Input: part model. Units: mm. Frame: model coordinates. A direction names the side the tool comes from. Coordinates: 2 decimals unless noted, no trailing zeros. Write each loop counter-clockwise with the first axis right and the second up, starting at its lowest first coordinate (ties: lowest second). Pieces come first, ordered by that corner, then holes.
from build123d import *

# Parameters (mm, degrees)
BOSS_EXTRUDE1_DEPTH     = 30
SKETCH2_W               = 30
SKETCH2_H               = 30
CUT_EXTRUDE1_DEPTH      = 30
CHAMFER1_SIZE           = 3
FILLET1_R               = 3
FILLET2_R               = 3
CUT_EXTRUDE2_DEPTH      = 30
CUT_EXTRUDE2_DEPTH_BACK = 30
SKETCH3_R               = 1.75
CUT_EXTRUDE3_DEPTH      = 50
CUT_EXTRUDE3_DEPTH_BACK = 30
SKETCH4_R               = 3
CUT_EXTRUDE4_DEPTH      = 88.933914818
CUT_EXTRUDE4_DEPTH_BACK = 88.933914818
SKETCH5_R               = 1.75


with BuildPart() as part:
    # Sketch1 → Boss-Extrude1 (new body)
    with BuildSketch(Plane(origin=(0, 0, 0), x_dir=(1, 0, 0), z_dir=(0, 1, 0))):
        Polygon((-65, 21.062445841), (-65, -21.062445841), (-21.005807434, -21.062445841), (-21.005807434, -30), (-15, -30), (-15, -21.062445841), (-36.062445841, 0), (-15, 21.062445841), (-15, 30), (-22, 30), (-22, 21.062445841), align=None)
    extrude(amount=BOSS_EXTRUDE1_DEPTH)

    # Sketch2 → Cut-Extrude1 (cut)
    with BuildSketch(Plane(origin=(0, 30, 0), x_dir=(1, 0, 0), z_dir=(0, 1, 0))):
        with Locations((-56.062445841, 0)):
            Rectangle(SKETCH2_W, SKETCH2_H)
    extrude(amount=-CUT_EXTRUDE1_DEPTH, mode=Mode.SUBTRACT)

    # Chamfer1
    chamfer1_edges = [part.edges().sort_by_distance(p)[0] for p in [
        (-21.005807434, 15, 21.062445841),
        (-22, 15, -21.062445841),
    ]]
    chamfer(chamfer1_edges, length=CHAMFER1_SIZE)

    # Fillet1
    fillet1_edges = [part.edges().sort_by_distance(p)[0] for p in [
        (-36.062445841, 15, 0),
        (-15, 15, 21.062445841),
        (-15, 15, -21.062445841),
        (-41.062445841, 15, 15),
        (-41.062445841, 15, -15),
    ]]
    fillet(fillet1_edges, radius=FILLET1_R)

    # Fillet2
    fillet2_edges = [part.edges().sort_by_distance(p)[0] for p in [
        (-15, 15, 30),
        (-21.005807434, 15, 30),
        (-65, 15, 21.062445841),
        (-65, 15, -21.062445841),
        (-22, 15, -30),
        (-15, 15, -30),
        (-65, 15, 15),
        (-65, 15, -15),
    ]]
    fillet(fillet2_edges, radius=FILLET2_R)

    # Sketch3 → Cut-Extrude2 (cut, two sides: drawn at the far end of the back side and taken through both)
    with BuildSketch(Plane.ZY.offset(22).offset(-CUT_EXTRUDE2_DEPTH_BACK)):
        with Locations(Location((-25, 15, 0), (0, 0, 57.605534529))):
            Circle(SKETCH3_R)
        with Locations(Location((25, 15, 0), (0, 0, 122.394465471))):
            Circle(SKETCH3_R)
    extrude(amount=CUT_EXTRUDE2_DEPTH + CUT_EXTRUDE2_DEPTH_BACK, mode=Mode.SUBTRACT)

    # Sketch4 → Cut-Extrude3 (cut, two sides: drawn at the far end of the back side and taken through both)
    with BuildSketch(Plane.XY.offset(-15).offset(-CUT_EXTRUDE3_DEPTH_BACK)):
        with Locations(Location((-55.062445841, 15.983841749, 0), (0, 0, 180))):
            Circle(SKETCH4_R)
    extrude(amount=CUT_EXTRUDE3_DEPTH + CUT_EXTRUDE3_DEPTH_BACK, mode=Mode.SUBTRACT)

    # Sketch5 → Cut-Extrude4 (cut, two sides: drawn at the far end of the back side and taken through both)
    with BuildSketch(Plane(origin=(0, 0, -21.062445841), x_dir=(-1, 0, 0), z_dir=(0, 0, -1)).offset(-CUT_EXTRUDE4_DEPTH_BACK)):
        with Locations((41, 15)):
            Circle(SKETCH5_R)
    extrude(amount=CUT_EXTRUDE4_DEPTH + CUT_EXTRUDE4_DEPTH_BACK, mode=Mode.SUBTRACT)


solid = part.part
Item 1: Section query A-A, the plane z = -25. Return loops of the section in (x, y), then the cut area to 4 significant figures.
Item 2: Access query for faces 5 (the face through (-21.006, 18, 26)), 6 (the face through (-15.222, 15.21, -21.172)), 7 (the face through (-43.3, 14.8, 14.9)). Directions: +Z, -Z, +X, -X, +Y, -Y. A direction counts if a zero-diameter tool reaches every point of the face in a straight line with its end or side. Return the directions, or none.
Item 3: Section query B-B, the plane x = -46. Return loops of the section in (y, z).
Item 4: Section query D-D, the plane z = 7.5. Return loops of the section in (x, y).
Item 5: Material intervals for line 1 (Z direction, x = -56.5, y = 28); line 2 (Y direction, x = -19.25, z = -25); line 3 (Z direction, x = -17, y = 15), sorted ascending.
Item 6: Pin query (flat end, axial travel): pin 1 Ø5 at (x, y) = (-57, 25.5) entering from -Z; pin 2 Ø8 at (x, z) = (-36, 13) entering from -Y; pin 3 Ø1.5 at (y, z) = (12, -11.5) entering from +X; pin 4 Ø8 at (x, z) = (-52.5, -8) entering from +Y. Return the tip coordinate at first contact, or that it passes through.
Item 7: Pull-direction query (Y, two-part tool) for faces 1 (the face through (-35, 0, 0)), 2 (the face through (-24.78, 14.79, 11.28)), 3 (the face through (-57.834, 17.133, 17.989)), 4 (the face through (-18.917, 14.85, -23.256)); classes: released by +Y, released by -Y, zero draft, split by the parting line, or undercut.
The answers:
1. outline: (-22, 0) - (-15, 0) - (-15, 13.25) - (-22, 13.25) - close; (-22, 16.75) - (-15, 16.75) - (-15, 30) - (-22, 30) - close
1. area: 185.5 mm2
2. face 5: +Z, -X, +Y, -Y
2. face 6: +X, +Y, -Y
2. face 7: -X, +Y, -Y
3. outline: (0, -21.06) - (30, -21.06) - (30, -15) - (0, -15) - close; (0, 15) - (30, 15) - (30, 21.06) - (0, 21.06) - close
4. outline: (-41.06, 0) - (-28.56, 0) - (-28.56, 30) - (-41.06, 30) - (-41.06, 16.75) arc R1.75 cw (long way) to (-41.06, 13.25) - close
5. line 1: z = -21.06 to -15, 15 to 21.06
5. line 2: y = 0 to 13.25, 16.75 to 30
5. line 3: z = -29.83 to -26.75, -23.25 to -19.06, 19.06 to 23.25, 26.75 to 29.83
6. pin 1: stops at z = -21.06
6. pin 2: stops at y = 0
6. pin 3: stops at x = -23.81
6. pin 4: passes through
7. face 1: released by -Y
7. face 2: zero draft
7. face 3: undercut
7. face 4: undercut
